Autodesk Inventor part; units mm, degrees
ref_plane "YZ Plane" through (0, 0, 0) normal (1, 0, 0) x (0, 1, 0)
ref_plane "XZ Plane" through (0, 0, 0) normal (0, 1, 0) x (-1, 0, 0)
ref_plane "XY Plane" through (0, 0, 0) normal (0, 0, 1) x (1, 0, 0)
sketch "Sketch1" plane through (0, 0, 0) normal (0, 0, 1) x (1, 0, 0)
  circle A0 centre (0, 0) radius 9.525
  circle A1 centre (0, -6.35) radius 1.5875
  circle A2 centre (0, 6.35) radius 1.5875
  line L0 (0, 9.525) -> (0, -9.525)
  dimension "d3" = 3.175
  dimension "d4" = 3.175
extrude "Extrusion2" add sketch "Sketch1" along normal blind 23.368
extrude "Extrusion3" cut sketch "Sketch1" along normal blind 6.35 contours L0 A2 | A2 L0 | L0 A1 | A1 L0
sketch "Sketch2" plane through (0, 0, 23.368) normal (0, 0, 1) x (1, 0, 0)
  circle A0 centre (0, 0) radius 9.525
  line L0 (0, 9.525) -> (0, -9.525)
  line L1 (0, 0) -> (25.4, 0) construction
  line L2 (0, 0) -> (25.4, 0) construction
  line L3 (8.2489, 4.7625) -> (-8.2489, -4.7625)
  line L4 (0, 0) -> (5.4993, 3.175)
  line L5 (5.4993, 3.175) -> (-5.4993, -3.175)
  circle A1 centre (-5.4993, -3.175) radius 1.5875
  circle A2 centre (5.4993, 3.175) radius 1.5875
  line L6 (0, 0) -> (15.1329, 0) construction
  line L7 (8.2489, 4.7625) -> (-8.2489, -4.7625)
  dimension "d22" = 6.35
  dimension "d23" = 12.7
  dimension "d24" = 3.175
  dimension "d25" = 3.175
extrude "Extrusion4" cut sketch "Sketch2" against normal blind 6.35 contours A2 L3 | L3 A2 | A1 L3 | L3 A1
properties part number "Crankshaft"
For this review, take the finished solid that the model builds, in its own axes (mm). A direction names the side the tool comes from. Give positions to 0.01 mm unless a question says otherwise; leave off trailing zeros. Write each loop counter-clockwise with the first axis right and the second up, starting at its lowest first coordinate (ties: lowest second). Pieces come first, ordered by that corner, then holes.
Item 1: Machinability: for faces 4 (the face through (-6, -3, 17.018)), 5 (the face through (0, 0, 0)), 6 (the face through (0.73, -4.94, 3.13)), which of the approach directions +Z, -Z, +X, -X, +Y, -Y give a long, thin tool a straight path to every point of the face, cutting with its end or side? Answer none if there is none.
Item 2: Take a section at B-B (y = 2). Give the boundary of the cut face in (x, z), and give its area (3 significant figures).
Item 3: Take a section at D-D (z = 20). Give the number of separate pieces and of enclosed holes in the cut face, and give its area (3 significant figures).
Item 4: Insertion check: P1, Ø5, axis at x = 4, z = 18, coming from the -Y side; P2, Ø6, axis at y = -3.5, z = 8, coming from the -X side; P3, Ø1.9, axis at x = 0, y = 6.35, coming from the -Z side. Each pin has a flat end and moves straight along its axis. Give the tip position at first contact, or say it passes through.
Item 5: The part is to be moulded in two halves that separate along Y. For faces 1 (the face through (-7.559, 5.796, 11.52)), 2 (the face through (-0.34, 7.9, 3.13)), 3 (the face through (0, 0, 23.368)), say which applies: +Y half, -Y half, draft (parallel to the pull), parting line (faces both ways), or undercut.
Item 6: Take a section at C-C (z = 14.25). Give the boundary of the cut face in (x, y) (3 decimals).
Item 7: Wall thickness on probe 1 along Y at (x, z) = (0, 4.25) (1 decimal); probe 2 along Z at (x, y) = (-1.5, 6); probe 3 along Y at (x, z) = (4.5, 19): over which ranges is each line inside the solid? List them lowest first.
Established:
1. face 4: +Z
1. face 5: -Z, +X, -X, +Y, -Y
1. face 6: -Z
2. outline: (-9.31, 0) - (9.31, 0) - (9.31, 23.37) - (6.57, 23.37) - (6.57, 17.02) - (4.43, 17.02) - (4.43, 23.37) - (-9.31, 23.37) - close
2. area: 422 mm2
3. separate pieces: 1
3. enclosed holes: 2
3. area: 269 mm2
4. P1: stops at y = -9.41
4. P2: stops at x = -9.51
4. P3: stops at z = 6.35
5. face 1: parting line
5. face 2: undercut
5. face 3: draft
6. outline: circle Ø19.05 at (0, 0)
7. probe 1: y = -9.5 to -7.9, -4.8 to 4.8, 7.9 to 9.5
7. probe 2: z = 6.35 to 23.37
7. probe 3: y = -8.39 to 1.94, 4.41 to 8.39
